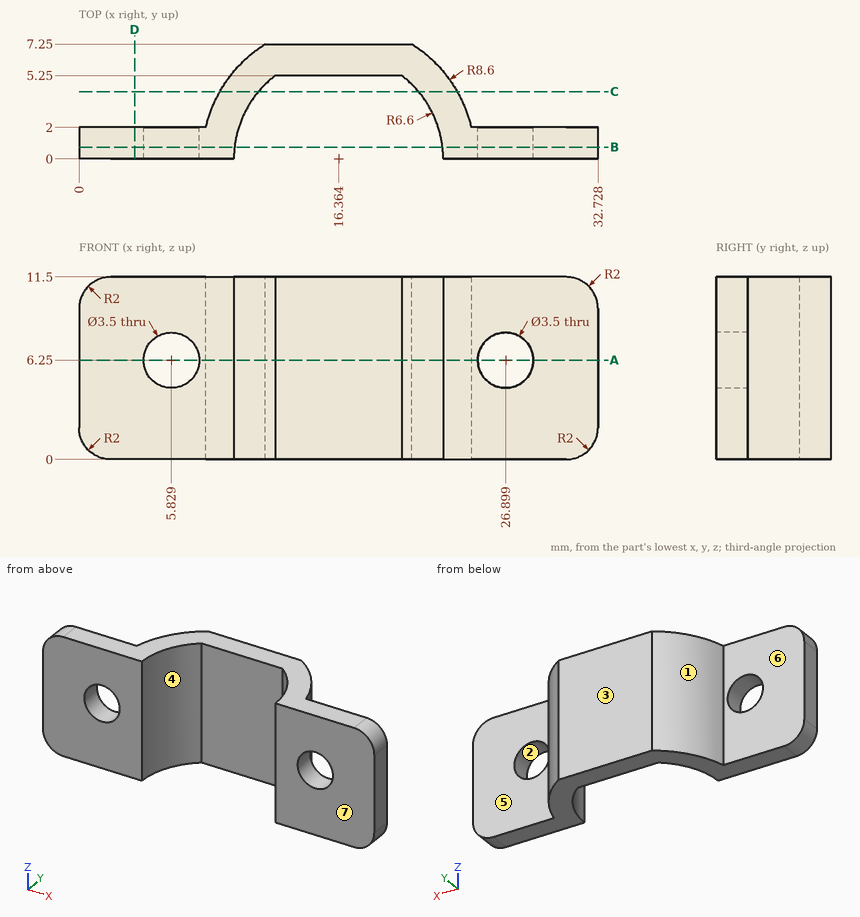
The drawing under review shows one solid part. Ordinate dimensions are in mm from its lowest x, y, z. A direction names the side the tool comes from. Give positions to 0.01 mm unless a question says otherwise; leave off trailing zeros. Loops run counter-clockwise (first coordinate to the right, second up) from the corner with the lowest first, then second, coordinate; pieces in that order, holes last. Notation, with made-up numbers: M 43,46.5 L 50,46.5 A27 cw 50,75.5 Z; hole C 36,80 d2. An arc over 180 degrees is marked long. One line per item, written item: value. Start each with the question number.
Q1. Add section C-C (y = 4.25). Give the boundary of the cut face in (x, z) (1 decimal).
Q2. Add section D-D (x = 3.5). Give the boundary of the cut face in (y, z), and give its area (3 significant figures).
Q3. Draft analysis for pull direction X (two halves, no side actions). For the marked faces 1, 2 and 3, state which applies: released by +X, released by -X, zero draft, split by the parting line, or undercut.
Q4. Clearance check with flat-ended pins moving along their axes: pin 1 Ø2.5 at (x, z) = (14.5, 5.5) entering from -Y; pin 2 Ø4 at (x, z) = (5.83, 6.25) entering from +Y; pin 3 Ø1.5 at (x, y) = (29, 4) entering from +Z. State where each tip first meets the part, or that it passes through.
Q5. Machinability: for the marked faces 4, 5, 6 and 7, which of the approach directions +Z, -Z, +X, -X, +Y, -Y give a long, thin tool a straight path to every point of the face, cutting with its end or side? Answer none if there is none.
Q6. Add section A-A (z = 6.25). Count the separate pieces of the cut face and the enclosed holes in it.
Q7. Add section B-B (y = 0.75). Give the boundary of the cut face in (x, z).
Q8. For L1, parallel to X at y = 1, z = 6.25; L2, parallel to Y at x = 4, z = 5.5; L3, parallel to Z at x = 28, y = 1.25, list the stretches that pass through material, from the lowest coordinate up.
Reply:
1. outline: M 8.9,0 L 11.3,0 L 11.3,11.5 L 8.9,11.5 Z; M 21.4,0 L 23.8,0 L 23.8,11.5 L 21.4,11.5 Z
2. outline: M 0,0 L 2,0 L 2,11.5 L 0,11.5 Z
2. area: 23.0 mm²
3. face 1: released by -X
3. face 2: undercut
3. face 3: zero draft
4. pin 1: y = 5.25
4. pin 2: y = 2
4. pin 3: through
5. face 4: +Z, -Z, -Y
5. face 5: +Z, -Z, +X, +Y
5. face 6: +Z, -Z, -X, +Y
5. face 7: +Z, -Z, +X, -X, -Y
6. separate pieces: 3
6. enclosed holes: 0
7. outline: M 0,2 A2 ccw 2,0 L 9.81,0 L 9.81,11.5 L 2,11.5 A2 ccw 0,9.5 Z; M 22.92,0 L 30.73,0 A2 ccw 32.73,2 L 32.73,9.5 A2 ccw 30.73,11.5 L 22.92,11.5 Z; hole C 5.83,6.25 d3.5; hole C 26.9,6.25 d3.5
8. L1: 0 to 4.08, 7.58 to 9.84, 22.89 to 25.15, 28.65 to 32.73
8. L2: 0 to 2
8. L3: 0 to 4.89, 7.61 to 11.5
